Check sheet for the modelled part. Datum: model origin and axes. Units: mm. A direction names the side the tool comes from. Round coordinates to 2 decimals unless told otherwise and drop trailing zeros. Write each loop counter-clockwise with the first axis right and the second up, starting at its lowest first coordinate (ties: lowest second). Pieces come first, ordered by that corner, then holes. Notation, with made-up numbers: (-13, -23.5) - (17, -23.5) arc R22 cw to (17, -11.5) - close; hole circle Ø2 at (23, 26.25). An arc over 180 degrees is marked (long way). Use one line per item in the form item = value. Start each with the question number.
1) Scan lines: probe 1 along Y at (x, z) = (23.5, -12); probe 2 along Z at (x, y) = (33, 6.25); probe 3 along Y at (x, z) = (-5, 34). Record each from-to range of solid material in increasing order.
2) Draft check along X on faces 5 (the face through (29.002, 6, 0)), 6 (the face through (-10, 10, -25)), 7 (the face through (35.002, 6, 0)). Enter one of: +X half, -X half, draft (parallel to the pull), parting line (faces both ways), or undercut.
3) Section check C-C (x = 0). Record the boundary of the cut face in (y, z).
4) Section check A-A (y = 5.75). Count the separate pieces of the cut face and the enclosed holes in it, then the cut area to 3 significant figures.
5) Section check D-D (x = 33.5). Record the boundary of the cut face in (y, z), then the cut area to 3 significant figures.
6) Gauge pin test, flat ends, axial feed: P1, Ø2.5, axis at x = 19.5, y = 4.5, coming from the +Z side; P2, Ø5.5, axis at y = 6, z = 27.5, coming from the +X side; P3, Ø3, axis at x = 33.5, y = 5, coming from the -Z side; P4, Ø25, axis at x = -20.5, z = 17, coming from the +Y side. Record the tip position at first contact, or that the pin passes through.
7) Set-up check for faces 1 (the face through (5, 6, -13)), 2 (the face through (32, 6, 3.204)), 3 (the face through (-20, 6, -12.5)), 4 (the face through (4.133, 5.698, 31.925)): record each of +Z, -Z, +X, -X, +Y, -Y from which the full face is reachable in a straight line by a thin tool's end or side.
8) Section check B-B (z = 0). Record the boundary of the cut face in (x, y), then the cut area to 3 significant figures.
from build123d import *

# Parameters (mm, degrees)
SKETCH1_R           = 42
BOSS_EXTRUDE1_DEPTH = 2
SKETCH2_R           = 3
SKETCH2_R_2         = 4
SKETCH2_R_3         = 4.5
SKETCH2_W           = 25
SKETCH2_H           = 25
SKETCH2_W_2         = 20
SKETCH2_H_2         = 20
SKETCH2_W_3         = 7
SKETCH2_H_3         = 7
SKETCH2_W_4         = 6
SKETCH2_H_4         = 6
BOSS_EXTRUDE2_DEPTH = 8
FILLET1_R           = 0.5


with BuildPart() as part:
    # Sketch1 → Boss-Extrude1 (new body)
    with BuildSketch(Plane(origin=(0, 0, 0), x_dir=(1, 0, 0), z_dir=(0, 1, 0))):
        Circle(SKETCH1_R)
    extrude(amount=BOSS_EXTRUDE1_DEPTH)

    # Sketch2 → Boss-Extrude2 (add)
    with BuildSketch(Plane(origin=(0, 2, 0), x_dir=(1, 0, 0), z_dir=(0, 1, 0))):
        with Locations((-20, 22.020171122)):
            Circle(SKETCH2_R)
        with Locations((-10.302496515, 25.377676752)):
            Circle(SKETCH2_R_2)
        with Locations((-20, -21.114457143)):
            Circle(SKETCH2_R_3)
        with Locations((5, -28.020526235)):
            Circle(SKETCH2_R_2)
        with Locations((-20, 0)):
            Rectangle(SKETCH2_W, SKETCH2_H)
        with Locations((15, 13.203564029)):
            Rectangle(SKETCH2_W_2, SKETCH2_H_2)
        with Locations((15, -13.203564029)):
            Rectangle(SKETCH2_W_2, SKETCH2_H_2)
        with Locations((-7.518218001, -28.243397592)):
            Rectangle(SKETCH2_W_3, SKETCH2_H_3)
        with Locations((32.002130678, -0.203564029)):
            Rectangle(SKETCH2_W_4, SKETCH2_H_4)
    extrude(amount=BOSS_EXTRUDE2_DEPTH)

    # Fillet1
    fillet1_edges = [part.edges().sort_by_distance(p)[0] for p in [
        (-23, 10, -22.020171122),
        (-14.302496515, 10, -25.377676752),
        (-24.5, 10, 21.114457143),
        (1, 10, 28.020526235),
        (-11.018218001, 10, 28.243397592),
        (-7.518218001, 10, 31.743397592),
        (-4.018218001, 10, 28.243397592),
        (-7.518218001, 10, 24.743397592),
        (35.002130678, 10, 0.203564029),
        (32.002130678, 10, -2.796435971),
        (29.002130678, 10, 0.203564029),
        (32.002130678, 10, 3.203564029),
    ]]
    fillet(fillet1_edges, radius=FILLET1_R)

    # Sketch6 → Revolve1 (revolve)
    with BuildSketch(Plane(origin=(0, 0, 0), x_dir=(0, 0, -1), z_dir=(1, 0, 0))):
        with BuildLine():
            Line((0, 0), (0, -15.408613296))
            ThreePointArc((0, -15.408613296), (-14.683539795, -11.247032644), (-25, 0))
            Line((-25, 0), (0, 0))
        make_face()
    revolve(axis=Axis((0, 0, 0), (0, -1, 0)))


solid = part.part
Results are:
q1.probe_1 = 0 to 10
q1.probe_2 = -2.8 to 3.2
q1.probe_3 = 0 to 2
q2.face_5 = undercut
q2.face_6 = draft
q2.face_7 = +X half
q3.outline = (0, -42) - (2, -42) - (2, 42) - (0, 42) - (0, 25) arc R27.99 ccw to (0, -25) - close
q4.separate_pieces = 9
q4.enclosed_holes = 0
q4.area = 1,700 mm²
q5.outline = (0, -25.33) - (2, -25.33) - (2, -2.8) - (9.5, -2.8) arc R0.5 ccw to (10, -2.3) - (10, 2.7) arc R0.5 ccw to (9.5, 3.2) - (2, 3.2) - (2, 25.33) - (0, 25.33) - close
q5.area = 149 mm²
q6.P1 = 23.2
q6.P2 = 9
q6.P3 = -2.8
q6.P4 = 10
q7.face_1 = -Z, +Y
q7.face_2 = +Z, +X, +Y
q7.face_3 = -X, +Y
q7.face_4 = +Y
q8.outline = (-42, 0) - (-25, 0) arc R27.99 ccw to (25, 0) - (42, 0) - (42, 2) - (35, 2) - (35, 9.5) arc R0.5 ccw to (34.5, 10) - (29.5, 10) arc R0.5 ccw to (29, 9.5) - (29, 2) - (-7.5, 2) - (-7.5, 10) - (-32.5, 10) - (-32.5, 2) - (-42, 2) - close
q8.area = 967 mm²
